The model under review builds one solid part; all positions refer to its coordinate system, in mm. Face numbers are marked on the shaded views. A direction names the side the tool comes from. Round coordinates to 2 decimals unless told otherwise and drop trailing zeros. Loops run counter-clockwise (first coordinate to the right, second up) from the corner with the lowest first, then second, coordinate; pieces in that order, holes last. Notation, with made-up numbers: (-14, 31.5) -> (23, 31.5) arc R24 ccw to (23, 53.5) -> close; hole circle Ø2 at (-19.75, 52.25). An arc over 180 degrees is marked (long way). Use a Markdown table: item, result. Add a question column.
1) Consider section A-A on z = -19.7. Give the boundary of the cut face in (x, y), plus the area to 3 significant figures.
2) Consider section C-C on z = -70. Give the boundary of the cut face in (x, y).
3) Insertion check: pin 1 (7 mm diameter, centred on x = 36, z = -145.5, fed in from -Y); pin 2 (2.5 mm diameter, centred on y = 6, z = -121, fed in from -X); pin 3 (4 mm diameter, centred on y = 5, z = -119.5, fed in from +X). Each pin has a flat end and moves straight along its axis. Give the tip position at first contact, or say it passes through.
4) For the marked faces 1, 2, 3, 4 and 5, list the 3-axis set-ups (+Z, -Z, +X, -X, +Y, -Y) from which the entire face can be reached by the end or side of a thin tool; tool diameter is ignored.
5) Mouldability with a two-part tool opening along Z and no side actions: class the marked faces 6 and 7 as released by +Z, released by -Z, zero draft, split by the parting line, or undercut.
6) Wall thickness on probe 1 along X at (y, z) = (8.75, -19.7); probe 2 along Z at (x, y) = (41.5, 10.75); probe 3 along Z at (x, y) = (33, 2.75): over which ranges is each line inside the solid? List them lowest first.
7) Consider section B-B on y = 10. State how many separate pieces and enclosed holes the cut face has, plus the area to 3 significant figures.
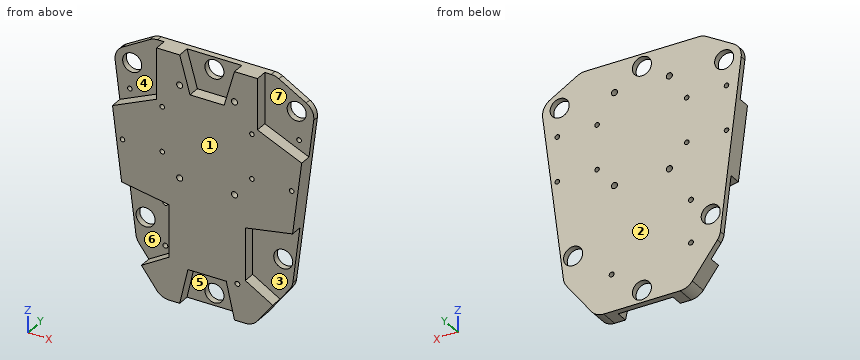
from build123d import *

# Parameters (mm, degrees)
SKETCH1_R           = 6.25
BOSS_EXTRUDE2_DEPTH = 12
SKETCH3_R           = 1.6
SKETCH3_R_2         = 2
SKETCH3_R_3         = 1.5
CUT_EXTRUDE3_DEPTH  = 194.554036966
SKETCH4_R           = 1.6
SKETCH4_R_2         = 6.25
SKETCH4_R_3         = 1.5
CUT_EXTRUDE4_DEPTH  = 8


with BuildPart() as part:
    # Sketch1 → Boss-Extrude2 (new body)
    with BuildSketch(Plane(origin=(0, 0, 0), x_dir=(1, 0, 0), z_dir=(0, 1, 0))):
        with BuildLine():
            Line((2.679491924, 0), (77.320508076, 0))
            ThreePointArc((77.320508076, 0), (79.908698527, 0.340741737), (82.320508076, 1.339745962))
            Line((82.320508076, 1.339745962), (100.238610908, 11.684767456))
            ThreePointArc((100.238610908, 11.684767456), (104.191551765, 15.890265607), (105.162092892, 21.579730085))
            Line((105.162092892, 21.579730085), (91.495098183, 131.422794828))
            ThreePointArc((91.495098183, 131.422794828), (90.837397635, 133.949109284), (89.548249395, 136.219116235))
            Line((89.548249395, 136.219116235), (73.056541302, 158.031029999))
            ThreePointArc((73.056541302, 158.031029999), (69.534663992, 160.952940857), (65.079908105, 162))
            Line((65.079908105, 162), (14.920091895, 162))
            ThreePointArc((14.920091895, 162), (10.465336008, 160.952940857), (6.943458698, 158.031029999))
            Line((6.943458698, 158.031029999), (-9.548249395, 136.219116235))
            ThreePointArc((-9.548249395, 136.219116235), (-10.837397635, 133.949109284), (-11.495098183, 131.422794828))
            Line((-11.495098183, 131.422794828), (-25.162092892, 21.579730085))
            ThreePointArc((-25.162092892, 21.579730085), (-24.191551765, 15.890265607), (-20.238610908, 11.684767456))
            Line((-20.238610908, 11.684767456), (-2.320508076, 1.339745962))
            ThreePointArc((-2.320508076, 1.339745962), (0.091301473, 0.340741737), (2.679491924, 0))
        make_face()
        with Locations(Location((-13.980762114, 20, 0), (0, 0, 270))):
            Circle(SKETCH1_R, mode=Mode.SUBTRACT)
        with Locations(Location((93.980762114, 19, 0), (0, 0, 270))):
            Circle(SKETCH1_R, mode=Mode.SUBTRACT)
        with Locations(Location((-5.164259013, 118.081783812, 0), (0, 0, 270))):
            Circle(SKETCH1_R, mode=Mode.SUBTRACT)
        with Locations(Location((85.164259013, 118.081783812, 0), (0, 0, 270))):
            Circle(SKETCH1_R, mode=Mode.SUBTRACT)
        with Locations(Location((40, 154, 0), (0, 0, 270))):
            Circle(SKETCH1_R, mode=Mode.SUBTRACT)
        with Locations(Location((40, 8, 0), (0, 0, 270))):
            Circle(SKETCH1_R, mode=Mode.SUBTRACT)
    extrude(amount=BOSS_EXTRUDE2_DEPTH)

    # Sketch3 → Cut-Extrude3 (cut, through all)
    with BuildSketch(Plane(origin=(0, 12, 0), x_dir=(1, 0, 0), z_dir=(0, 1, 0))):
        with Locations(Location((7.799462252, 104.803453548, 0), (0, 0, 270))):
            Circle(SKETCH3_R)
        with Locations(Location((7.799462252, 132.743453548, 0), (0, 0, 270))):
            Circle(SKETCH3_R)
        with Locations(Location((59.869462252, 137.823453548, 0), (0, 0, 270))):
            Circle(SKETCH3_R)
        with Locations(Location((58, 19.7, 0), (0, 0, 270))):
            Circle(SKETCH3_R_2)
        with Locations(Location((22, 19.7, 0), (0, 0, 90))):
            Circle(SKETCH3_R_2)
        with Locations(Location((22, 80.3, 0), (0, 0, 270))):
            Circle(SKETCH3_R_2)
        with Locations(Location((58, 80.3, 0), (0, 0, 90))):
            Circle(SKETCH3_R_2)
        with Locations(Location((10.577199901, 37.314321378, 0), (0, 0, 270))):
            Circle(SKETCH3_R_3)
        with Locations(Location((-15.522800099, 66.494321378, 0), (0, 0, 270))):
            Circle(SKETCH3_R_3)
        with Locations(Location((-15.522800099, 37.314321378, 0), (0, 0, 270))):
            Circle(SKETCH3_R_3)
        with Locations(Location((10.577199901, 66.494321378, 0), (0, 0, 270))):
            Circle(SKETCH3_R_3)
        with Locations(Location((95.522800099, 37.314321378, 0), (0, 0, 90))):
            Circle(SKETCH3_R_3)
        with Locations(Location((95.522800099, 66.494321378, 0), (0, 0, 90))):
            Circle(SKETCH3_R_3)
        with Locations(Location((69.422800099, 37.314321378, 0), (0, 0, 90))):
            Circle(SKETCH3_R_3)
        with Locations(Location((69.422800099, 66.494321378, 0), (0, 0, 90))):
            Circle(SKETCH3_R_3)
    extrude(amount=-CUT_EXTRUDE3_DEPTH, mode=Mode.SUBTRACT)

    # Sketch4 → Cut-Extrude4 (cut)
    # profile 1 of 8: a face of its own
    with BuildSketch(Plane.XZ):
        with BuildLine():
            Line((14.920091895, -99.763149928), (-16.111032357, -94.324049484))
            Line((-16.111032357, -94.324049484), (-11.495098183, -131.422794828))
            ThreePointArc((-11.495098183, -131.422794828), (-10.837397635, -133.949109284), (-9.548249395, -136.219116235))
            Line((-9.548249395, -136.219116235), (-3.07018894, -144.786991388))
            Line((-3.07018894, -144.786991388), (14.920091895, -134.081783812))
            Line((14.920091895, -134.081783812), (14.920091895, -99.763149928))
        make_face()
        with Locations(Location((7.799462252, -132.743453548, 0), (0, 0, 90))):
            Circle(SKETCH4_R, mode=Mode.SUBTRACT)
        with Locations(Location((-5.164259013, -118.081783812, 0), (0, 0, 270))):
            Circle(SKETCH4_R_2, mode=Mode.SUBTRACT)
        with Locations(Location((7.799462252, -104.803453548, 0), (0, 0, 90))):
            Circle(SKETCH4_R, mode=Mode.SUBTRACT)
    # profile 2 of 8: a face of its own
    with BuildSketch(Plane.XZ):
        with BuildLine():
            Line((52.588445494, -138.333140663), (40, -138.333140663))
            Line((40, -138.333140663), (40, -147.75))
            ThreePointArc((40, -147.75), (44.419417382, -149.580582618), (46.25, -154))
            ThreePointArc((46.25, -154), (44.419417382, -158.419417382), (40, -160.25))
            Line((40, -160.25), (40, -162))
            Line((40, -162), (57.978215662, -162))
            Line((57.978215662, -162), (52.588445494, -138.333140663))
        make_face()
    # profile 3 of 8: a face of its own
    with BuildSketch(Plane.XZ):
        with BuildLine():
            Line((40, -147.75), (40, -138.333140663))
            Line((40, -138.333140663), (27.411554506, -138.333140663))
            Line((27.411554506, -138.333140663), (22.021784338, -162))
            Line((22.021784338, -162), (40, -162))
            Line((40, -162), (40, -160.25))
            ThreePointArc((40, -160.25), (33.75, -154), (40, -147.75))
        make_face()
    # profile 4 of 8: a face of its own
    with BuildSketch(Plane.XZ):
        with BuildLine():
            Line((91.495098183, -131.422794828), (96.111032357, -94.324049484))
            Line((96.111032357, -94.324049484), (65.079908105, -99.763149928))
            Line((65.079908105, -99.763149928), (65.079908105, -134.081783812))
            Line((65.079908105, -134.081783812), (83.07018894, -144.786991388))
            Line((83.07018894, -144.786991388), (89.548249395, -136.219116235))
            ThreePointArc((89.548249395, -136.219116235), (90.837397635, -133.949109284), (91.495098183, -131.422794828))
        make_face()
        with Locations(Location((85.164259013, -118.081783812, 0), (0, 0, 270))):
            Circle(SKETCH4_R_2, mode=Mode.SUBTRACT)
    # profile 5 of 8: a face of its own
    with BuildSketch(Plane.XZ):
        with BuildLine():
            Line((100.238610908, -11.684767456), (82.320508076, -1.339745962))
            ThreePointArc((82.320508076, -1.339745962), (79.908698527, -0.340741737), (77.320508076, 0))
            Line((77.320508076, 0), (73.056541302, 0))
            Line((73.056541302, 0), (73.056541302, -33.441212659))
            Line((73.056541302, -33.441212659), (102.077468862, -46.371175776))
            Line((102.077468862, -46.371175776), (105.162092892, -21.579730085))
            ThreePointArc((105.162092892, -21.579730085), (104.191551765, -15.890265607), (100.238610908, -11.684767456))
        make_face()
        with Locations(Location((95.522800099, -37.314321378, 0), (0, 0, 270))):
            Circle(SKETCH4_R_3, mode=Mode.SUBTRACT)
        with Locations(Location((93.980762114, -19, 0), (0, 0, 270))):
            Circle(SKETCH4_R_2, mode=Mode.SUBTRACT)
    # profile 6 of 8: a face of its own
    with BuildSketch(Plane.XZ):
        with BuildLine():
            Line((51.192803455, -24.002493724), (57.978215662, 0))
            Line((57.978215662, 0), (40, 0))
            Line((40, 0), (40, -1.75))
            ThreePointArc((40, -1.75), (44.419417382, -3.580582618), (46.25, -8))
            ThreePointArc((46.25, -8), (44.419417382, -12.419417382), (40, -14.25))
            Line((40, -14.25), (40, -24.002493724))
            Line((40, -24.002493724), (51.192803455, -24.002493724))
        make_face()
    # profile 7 of 8: a face of its own
    with BuildSketch(Plane.XZ):
        with BuildLine():
            Line((40, -1.75), (40, 0))
            Line((40, 0), (22.021784338, 0))
            Line((22.021784338, 0), (28.807196545, -24.002493724))
            Line((28.807196545, -24.002493724), (40, -24.002493724))
            Line((40, -24.002493724), (40, -14.25))
            ThreePointArc((40, -14.25), (33.75, -8), (40, -1.75))
        make_face()
    # profile 8 of 8: a face of its own
    with BuildSketch(Plane.XZ):
        with BuildLine():
            Line((6.943458698, -33.441212659), (6.943458698, 0))
            Line((6.943458698, 0), (2.679491924, 0))
            ThreePointArc((2.679491924, 0), (0.091301473, -0.340741737), (-2.320508076, -1.339745962))
            Line((-2.320508076, -1.339745962), (-20.238610908, -11.684767456))
            ThreePointArc((-20.238610908, -11.684767456), (-24.191551765, -15.890265607), (-25.162092892, -21.579730085))
            Line((-25.162092892, -21.579730085), (-22.077468862, -46.371175776))
            Line((-22.077468862, -46.371175776), (6.943458698, -33.441212659))
        make_face()
        with Locations(Location((-15.522800099, -37.314321378, 0), (0, 0, 90))):
            Circle(SKETCH4_R_3, mode=Mode.SUBTRACT)
        with Locations(Location((-13.980762114, -20, 0), (0, 0, 270))):
            Circle(SKETCH4_R_2, mode=Mode.SUBTRACT)
    extrude(amount=-CUT_EXTRUDE4_DEPTH, mode=Mode.SUBTRACT)


solid = part.part
Result set:
| question | item | result |
|---|---|---|
| 1 | outline | (-25.22, 8) -> (-20.22, 8) -> (-20.22, 12) -> (-25.22, 12) -> close; (-7.74, 8) -> (6.94, 8) -> (6.94, 0) -> (20, 0) -> (20, 12) -> (-7.74, 12) -> close; (24, 0) -> (27.59, 0) -> (27.59, 8) -> (52.41, 8) -> (52.41, 0) -> (56, 0) -> (56, 12) -> (24, 12) -> close; (60, 0) -> (73.06, 0) -> (73.06, 8) -> (87.77, 8) -> (87.77, 12) -> (60, 12) -> close; (100.19, 8) -> (105.22, 8) -> (105.22, 12) -> (100.19, 12) -> close |
| 1 | area | 656 mm2 |
| 2 | outline | (-19.14, 0) -> (99.14, 0) -> (99.14, 12) -> (-19.14, 12) -> close |
| 3 | pin 1 | y = 8 |
| 3 | pin 2 | x = 14.92 |
| 3 | pin 3 | x = 65.08 |
| 4 | face 1 | +Z, -Z, +X, -X, -Y |
| 4 | face 2 | +Z, -Z, +X, -X, +Y |
| 4 | face 3 | +X, -Y |
| 4 | face 4 | +Z, -X, -Y |
| 4 | face 5 | -Z, -Y |
| 5 | face 6 | undercut |
| 5 | face 7 | zero draft |
| 6 | probe 1 | -25.22 to -20.22, -7.74 to 20, 24 to 56, 60 to 87.77, 100.19 to 105.22 |
| 6 | probe 2 | -162 to -160.07, -147.93 to -14.07, -1.93 to 0 |
| 6 | probe 3 | -138.33 to -24 |
| 7 | separate pieces | 1 |
| 7 | enclosed holes | 21 |
| 7 | area | 16,900 mm2 |
